Autodesk Inventor part; units mm, degrees
ref_plane "YZ Plane" through (0, 0, 0) normal (1, 0, 0) x (0, 1, 0)
ref_plane "XZ Plane" through (0, 0, 0) normal (0, 1, 0) x (-1, 0, 0)
ref_plane "XY Plane" through (0, 0, 0) normal (0, 0, 1) x (1, 0, 0)
sketch "スケッチ1" plane through (0, 0, 0) normal (1, 0, 0) x (0, 1, 0)
  circle A0 centre (0, 0) radius 11
  dimension "d0" = 22
extrude "押し出し1" add sketch "スケッチ1" along normal blind 6
sketch "スケッチ2" plane through (0, 0, 0) normal (-1, 0, 0) x (0, 0, 1)
  circle A0 centre (0, 0) radius 9.5
  circle A1 centre (0, 0) radius 11
  dimension "d3" = 19
  dimension "d4" = 22
extrude "押し出し2" cut sketch "スケッチ2" against normal blind 4.5
sketch "スケッチ3" plane through (0, 0, 0) normal (-1, 0, 0) x (0, 0, 1)
  circle A0 centre (0, 0) radius 4
  dimension "d7" = 8
extrude "押し出し3" cut sketch "スケッチ3" against normal through all
properties part number "8mmベアリング"
Geometry: final body of the model. Coordinates: model frame, mm. A direction names the side the tool comes from. Round coordinates to 2 decimals unless told otherwise and drop trailing zeros. Order: outer loops, then holes, each group sorted by start corner. A loop starts at its lowest first (then second) coordinate and runs counter-clockwise, first axis right, second up. Notation, with made-up numbers: (81, 11) -> (129, 11) arc R11 cw to (129, 24) -> close; hole circle Ø8 at (48, 81.5). An arc over 180 degrees is marked (long way). Write each question's results on one line, items separated by ' | '.
Q1. Ray query, line 1 along Y through (x, z) = (1.65, 0); line 2 along Y through (x, z) = (5.25, -2.25); line 3 along Z through (x, y) = (0.55, -0.25). Return the intervals inside material, ascending.
Response values:
line 1: -9.5 to -4, 4 to 9.5 | line 2: -10.77 to -3.31, 3.31 to 10.77 | line 3: -9.5 to -3.99, 3.99 to 9.5
Q2. Section query A-A (z = 0). Output: boundary loops of the cut face in (x, y), and give its area (3 significant figures).
Response values:
outline: (0, -9.5) -> (4.5, -9.5) -> (4.5, -11) -> (6, -11) -> (6, -4) -> (0, -4) -> close; (0, 4) -> (6, 4) -> (6, 11) -> (4.5, 11) -> (4.5, 9.5) -> (0, 9.5) -> close | area: 70.5 mm²
Q3. Access query for faces 1 (the face through (2.22, -8.43, 4.38)), 2 (the face through (6, 0, -5)). Directions: +Z, -Z, +X, -X, +Y, -Y. A direction counts if a zero-diameter tool reaches every point of the face in a straight line with its end or side. Return the directions, or none.
Response values:
face 1: -X | face 2: +Z, -Z, +X, +Y, -Y
Q4. Section query D-D (y = 8). Output: boundary loops of the cut face in (x, z).
Response values:
outline: (0, -5.12) -> (4.5, -5.12) -> (4.5, -7.55) -> (6, -7.55) -> (6, 7.55) -> (4.5, 7.55) -> (4.5, 5.12) -> (0, 5.12) -> close
Q5. Pin query (flat end, axial travel): pin 1 Ø2 at (x, z) = (1.5, 4.5) entering from -Y; pin 2 Ø1.5 at (x, y) = (5.5, 4) entering from +Z; pin 3 Ø2 at (x, z) = (2.5, 5) entering from -Y; pin 4 Ø1.5 at (y, z) = (-1, 7.5) entering from -X. Return the tip coordinate at first contact, or that it passes through.
Response values:
pin 1: y = -8.83 | pin 2: z = 10.51 | pin 3: y = -8.62 | pin 4: x = 0
Q6. Section query C-C (x = 5.5). Output: boundary loops of the cut face in (y, z), and give its area (3 significant figures).
Response values:
outline: circle Ø22 at (0, 0); hole circle Ø8 at (0, 0) | area: 330 mm²
Q7. Pull-direction query (Z, two-part tool) for faces 3 (the face through (4.5, 0, -10)), 4 (the face through (2.958, -3.905, -0.867)), 5 (the face through (5.24, -2.38, 10.74)); classes: released by +Z, released by -Z, zero draft, split by the parting line, or undercut.
Response values:
face 3: zero draft | face 4: undercut | face 5: split by the parting line
